Design review of the part built by this model. Coordinates are the model's own, in mm. Coordinates: 2 decimals unless noted, no trailing zeros. Write each loop counter-clockwise with the first axis right and the second up, starting at its lowest first coordinate (ties: lowest second). Pieces come first, ordered by that corner, then holes. Notation, with made-up numbers: M -22,23 L 0,23 A13 cw 0,38 Z; hole C 86,42 d10. An arc over 180 degrees is marked long. Write item = value, one per line.
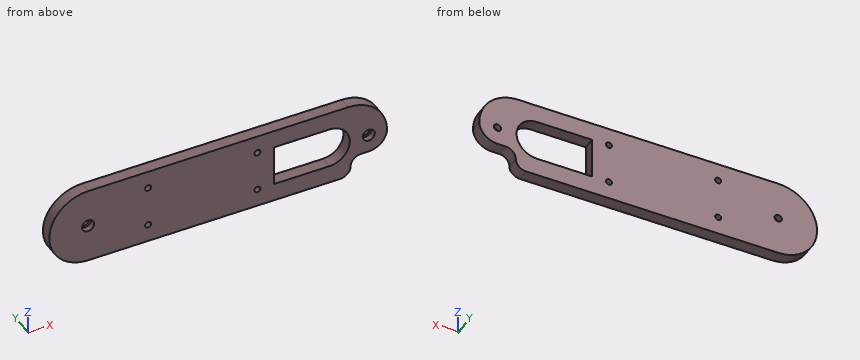
```python
from build123d import *

# Parameters (mm, degrees)
F0_R     = 3.175
F0_R_2   = 6.35
F1_DEPTH = 12.7
F2_DEPTH = 6.35
F0_R_3   = 3.81
F3_DEPTH = 6.35


with BuildPart() as f1:
    # F0 (on Front) → F1 (new body)
    with BuildSketch(Plane.XZ):
        with BuildLine():
            ThreePointArc((-140.4550125721, -108.3747648736), (-137.293230275, -100.7415471707), (-129.6600125721, -97.5797648736))
            Line((-129.6600125721, -97.5797648736), (-122.9925125721, -97.5797648736))
            Line((-122.9925125721, -97.5797648736), (-121.4050125721, -97.5797648736))
            ThreePointArc((-121.4050125721, -97.5797648736), (-107.9346283905, -92.0001490552), (-102.3550125721, -78.5297648736))
            ThreePointArc((-102.3550125721, -78.5297648736), (-114.2581929847, -49.7929452862), (-142.9950125721, -37.8897648736))
            Line((-142.9950125721, -37.8897648736), (-150.1512528809, -37.8897648736))
            Line((-150.1512528809, -37.8897648736), (-415.0925125721, -37.8897648736))
            Line((-415.0925125721, -37.8897648736), (-415.0925125721, -72.1797648736))
            ThreePointArc((-415.0925125721, -72.1797648736), (-410.6023845116, -74.0396368131), (-408.7425125721, -78.5297648736))
            ThreePointArc((-408.7425125721, -78.5297648736), (-410.6023845116, -83.0198929341), (-415.0925125721, -84.8797648736))
            Line((-415.0925125721, -84.8797648736), (-415.0925125721, -119.1697648736))
            Line((-415.0925125721, -119.1697648736), (-151.2500125721, -119.1697648736))
            ThreePointArc((-151.2500125721, -119.1697648736), (-143.6167948692, -116.0079825765), (-140.4550125721, -108.3747648736))
        make_face()
        with Locations((-352.2111295721, -100.1197648736)):
            Circle(F0_R, mode=Mode.SUBTRACT)
        with Locations((-237.9111295721, -100.1197648736)):
            Circle(F0_R, mode=Mode.SUBTRACT)
        with BuildLine():
            ThreePointArc((-162.8412207992, -56.9397648736), (-141.2512207992, -78.5297648736), (-162.8412207992, -100.1197648736))
            Line((-162.8412207992, -100.1197648736), (-220.3693254323, -100.1197648736))
            Line((-220.3693254323, -100.1197648736), (-220.3693254323, -56.9397648736))
            Line((-220.3693254323, -56.9397648736), (-162.8412207992, -56.9397648736))
        make_face(mode=Mode.SUBTRACT)
        with Locations((-121.4050125721, -78.5297648736)):
            Circle(F0_R_2, mode=Mode.SUBTRACT)
        with Locations((-352.2111295721, -56.9397648736)):
            Circle(F0_R, mode=Mode.SUBTRACT)
        with Locations((-237.9111295721, -56.9397648736)):
            Circle(F0_R, mode=Mode.SUBTRACT)
        with BuildLine():
            ThreePointArc((-415.0925125721, -37.8897648736), (-455.7325125721, -78.5297648736), (-415.0925125721, -119.1697648736))
            Line((-415.0925125721, -119.1697648736), (-415.0925125721, -84.8797648736))
            ThreePointArc((-415.0925125721, -84.8797648736), (-421.4425125721, -78.5297648736), (-415.0925125721, -72.1797648736))
            Line((-415.0925125721, -72.1797648736), (-415.0925125721, -37.8897648736))
        make_face()
    extrude(amount=F1_DEPTH)

    # F0 (on Front) → F2 (join)
    with BuildSketch(Plane.XZ):
        with BuildLine():
            ThreePointArc((-415.0925125721, -72.1797648736), (-421.4425125721, -78.5297648736), (-415.0925125721, -84.8797648736))
            Line((-415.0925125721, -84.8797648736), (-415.0925125721, -82.3397648736))
            ThreePointArc((-415.0925125721, -82.3397648736), (-418.9025125721, -78.5297648736), (-415.0925125721, -74.7197648736))
            Line((-415.0925125721, -74.7197648736), (-415.0925125721, -72.1797648736))
        make_face()
        with BuildLine():
            Line((-415.0925125721, -82.3397648736), (-415.0925125721, -84.8797648736))
            ThreePointArc((-415.0925125721, -84.8797648736), (-410.6023845116, -83.0198929341), (-408.7425125721, -78.5297648736))
            ThreePointArc((-408.7425125721, -78.5297648736), (-410.6023845116, -74.0396368131), (-415.0925125721, -72.1797648736))
            Line((-415.0925125721, -72.1797648736), (-415.0925125721, -74.7197648736))
            ThreePointArc((-415.0925125721, -74.7197648736), (-412.3984357358, -75.8356880373), (-411.2825125721, -78.5297648736))
            ThreePointArc((-411.2825125721, -78.5297648736), (-412.3984357358, -81.2238417099), (-415.0925125721, -82.3397648736))
        make_face()
    extrude(amount=F2_DEPTH)

    # F0 (on Front) → F3 (join)
    with BuildSketch(Plane.XZ):
        with Locations((-121.4050125721, -78.5297648736)):
            Circle(F0_R_2)
        with Locations((-121.4050125721, -78.5297648736)):
            Circle(F0_R_3, mode=Mode.SUBTRACT)
    extrude(amount=F3_DEPTH)


solid = f1.part
```
Q1. Wall thickness on line 1 (X direction, y = -6, z = -77); line 2 (Z direction, x = -179.5, y = -2.5); line 3 (X direction, y = -8.75, z = -80): over which ranges is each line inside the solid? List them lowest first.
Check result:
line_1 = -455.7 to -418.58, -411.6 to -220.37, -141.31 to -124.89, -117.92 to -102.38
line_2 = -119.17 to -100.12, -56.94 to -37.89
line_3 = -455.71 to -421.27, -408.92 to -220.37, -141.3 to -127.58, -115.23 to -102.41
Q2. For P1, Ø10, axis at x = -275, z = -47.5, coming from the +Y side; P2, Ø3, axis at y = -1.5, z = -87.5, coming from the -X side; P3, Ø9, axis at x = -121.41, z = -78.53, coming from the -Y side, all flat-tipped, find the tip position at first contact; note any pin that passes through.
Check result:
P1 = 0
P2 = -455.04
P3 = -6.35
Q3. Consider section B-B, the plane z = -94. State the section outline as (x, y) points.
Check result:
outline = M -452.67,-12.7 L -220.37,-12.7 L -220.37,0 L -452.67,0 Z; M -147.78,-12.7 L -110.29,-12.7 L -110.29,0 L -147.78,0 Z
Q4. Consider section A-A, the plane y = -3. State the section outline as (x, z) points (3 decimals).
Check result:
outline = M -415.093,-119.17 L -151.25,-119.17 A10.795 ccw -140.455,-108.375 A10.795 cw -129.66,-97.58 L -121.405,-97.58 A19.05 ccw -102.355,-78.53 A40.64 ccw -142.995,-37.89 L -415.093,-37.89 A40.64 ccw Z; hole C -415.093,-78.53 d7.62; hole C -352.211,-100.12 d6.35; hole C -352.211,-56.94 d6.35; hole C -237.911,-100.12 d6.35; hole C -237.911,-56.94 d6.35; hole M -220.369,-100.12 L -162.841,-100.12 A21.59 ccw -162.841,-56.94 L -220.369,-56.94 Z; hole C -121.405,-78.53 d7.62
